Geometry: see drawing. Coordinates: mm, zero at the bounding-box minimum. A direction names the side the tool comes from. Round coordinates to 2 decimals unless told otherwise and drop trailing zeros. Loops run counter-clockwise (first coordinate to the right, second up) from the corner with the lowest first, then second, coordinate; pieces in that order, holes last. Notation, with made-up numbers: (64.25, -20) - (86.25, -20) arc R13 ccw to (86.25, -10) - close; hole circle Ø5 at (40, 5). An arc over 180 degrees is marked (long way). Use CSV: the item, a comma, the result in double quotes.
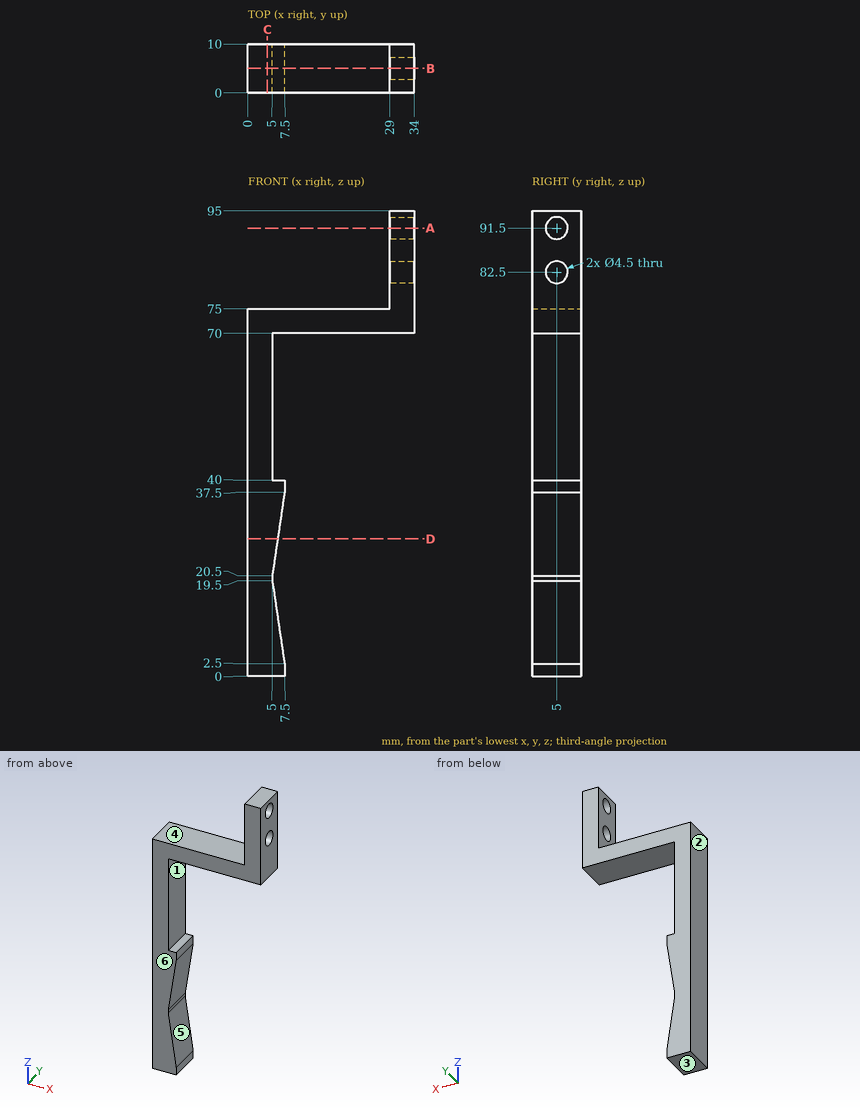
Item 1: Pin query (flat end, axial travel): P1, Ø0.8, axis at y = 6, z = 38, coming from the +X side; P2, Ø3, axis at x = 16, y = 9, coming from the +Z side; P3, Ø1, axis at y = 3, z = 29, coming from the +X side; P4, Ø2.5, axis at y = 5, z = 91.5, coming from the +X side. Return the tip coordinate at first contact, or that it passes through.
Final values:
P1,"stops at x = 7.5"
P2,"stops at z = 75"
P3,"stops at x = 6.32"
P4,"passes through"
Item 2: Mould query, pull axis Z, two halves, no side actions, for the marked faces 3, 4, 5 and 6. Classes: released by +Z, released by -Z, zero draft, split by the parting line, or undercut.
Final values:
face 3,"released by -Z"
face 4,"released by +Z"
face 5,"undercut"
face 6,"zero draft"
Item 3: Section C-C on x = 4. Return the cut outline in (y, z), plus the area to 3 significant figures.
Final values:
outline,"(0, 0) - (10, 0) - (10, 75) - (0, 75) - close"
area,"750 mm²"
Item 4: Section D-D on z = 28. Return the cut outline in (x, y), plus the area to 3 significant figures.
Final values:
outline,"(0, 0) - (6.1, 0) - (6.1, 10) - (0, 10) - close"
area,"61.0 mm²"
Item 5: Section A-A on z = 91.5. Return the cut outline in (x, y).
Final values:
outline,"(29, 0) - (34, 0) - (34, 2.75) - (29, 2.75) - close; (29, 7.25) - (34, 7.25) - (34, 10) - (29, 10) - close"
Item 6: Section B-B on y = 5. Return the cut outline in (x, z), plus the area to 3 significant figures.
Final values:
outline,"(0, 0) - (7.5, 0) - (7.5, 2.5) - (5, 19.5) - (5, 20.5) - (7.5, 37.5) - (7.5, 40) - (5, 40) - (5, 70) - (34, 70) - (34, 80.25) - (29, 80.25) - (29, 75) - (0, 75) - close; (29, 84.75) - (34, 84.75) - (34, 89.25) - (29, 89.25) - close; (29, 93.75) - (34, 93.75) - (34, 95) - (29, 95) - close"
area,"630 mm²"
Item 7: Material intervals for line 1 (Y direction, x = 30.6, z = 82.5); line 2 (Z direction, x = 8.5, y = 2.75); line 3 (X direction, y = 1.5, z = 91), sorted ascending.
Final values:
line 1,"y = 0 to 2.75, 7.25 to 10"
line 2,"z = 70 to 75"
line 3,"x = 29 to 34"
Item 8: Reachability of the marked faces 1 and 2 from +Z, -Z, +X, -X, +Y, -Y: full face, straight path, thin tool, end or side. Return the list, or none.
Final values:
face 1,"+X, +Y, -Y"
face 2,"+Z, -Z, -X, +Y, -Y"
